Part model, mm, in its own coordinate system. Round coordinates to 2 decimals unless told otherwise and drop trailing zeros. Write each loop counter-clockwise with the first axis right and the second up, starting at its lowest first coordinate (ties: lowest second). Pieces come first, ordered by that corner, then holes. Notation, with made-up numbers: (9.25, -28) -> (16.25, -28) arc R6 cw to (16.25, -22) -> close; hole circle Ø7 at (88.25, 63). An arc over 180 degrees is marked (long way). Return JSON: item names as keys, results as strings. Group by question number.
(1) Drop a flat-ended pin along its axis: pin 1 Ø5 at (y, z) = (-2.5, 61.5) entering from -X. Give the stop position or say it passes through.
(2) Drill centre lines: L1, parallel to Z at x = 0, y = -6; L2, parallel to Z at x = 9, y = -7.5; L3, parallel to X at y = -2.75, z = 17. Where is each one in solid material? Low to high. Write a range as from..to.
(3) Saw through at C-C (x = 0). List the corners of the cut face in (y, z), plus the area to 3 significant figures.
(4) Saw through at B-B (y = -3.5). List the corners of the cut face in (x, z), plus the area to 3 significant figures.
(5) Saw through at D-D (x = -39). List the corners of the cut face in (y, z), plus the area to 3 significant figures.
(6) Saw through at A-A (z = 0). List the corners of the cut face in (x, y).
from build123d import *

# Parameters (mm, degrees)
F0_W     = 150
F0_H     = 200
F1_DEPTH = 10
F2_R     = 50
F4_D     = 50


with BuildPart() as f1:
    # F0 (on Front) → F1 (new body)
    with BuildSketch(Plane.XZ):
        Rectangle(F0_W, F0_H)
    extrude(amount=F1_DEPTH)

    # F2
    f2_edges = [f1.edges().sort_by_distance(p)[0] for p in [
        (-75, -5, 100),
        (-75, -5, -100),
    ]]
    fillet(f2_edges, radius=F2_R)

    # F4 (through all)
    with Locations(Plane(origin=(0, 0, 0), x_dir=(1, 0, 0), z_dir=(0, 1, 0))):
        with Locations((0, 0)):
            Hole(F4_D / 2)


solid = f1.part
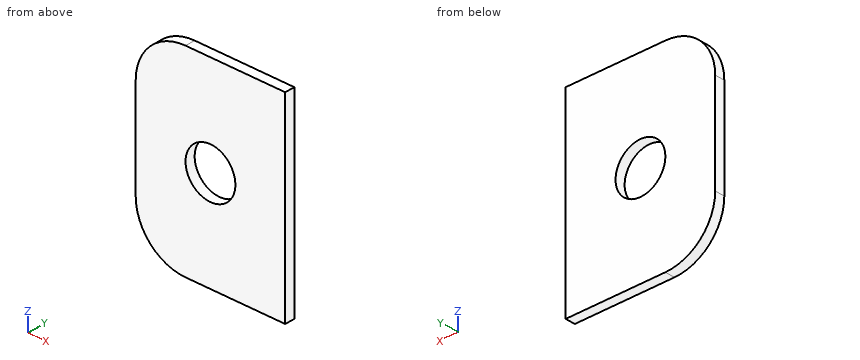
Computed values:
{
 "1": {"pin 1": "x = -74.18"},
 "2": {"L1": "-100..-25, 25..100", "L2": "-100..-23.32, 23.32..100", "L3": "-75..-18.33, 18.33..75"},
 "3": {"outline": "(-10, -100) -> (0, -100) -> (0, -25) -> (-10, -25) -> close; (-10, 25) -> (0, 25) -> (0, 100) -> (-10, 100) -> close", "area": "1,500 mm2"},
 "4": {"outline": "(-75, -50) arc R50 ccw to (-25, -100) -> (75, -100) -> (75, 100) -> (-25, 100) arc R50 ccw to (-75, 50) -> close; hole circle Ø50 at (0, 0)", "area": "27,000 mm2"},
 "5": {"outline": "(-10, -98) -> (0, -98) -> (0, 98) -> (-10, 98) -> close", "area": "1,960 mm2"},
 "6": {"outline": "(-75, -10) -> (-25, -10) -> (-25, 0) -> (-75, 0) -> close; (25, -10) -> (75, -10) -> (75, 0) -> (25, 0) -> close"}
}
